```python
from build123d import *

# Parameters (mm, degrees)
EXTRUDE_1_DEPTH       = 2
HOLE_WIZARD_4_0_4_1_D = 4
HOLE_WIZARD_4_0_4_2_D = 4
FILLET_1_R            = 5
FILLET_2_R            = 5


with BuildPart() as part:
    # 草圖1 → 填料-伸長1 (new body)
    with BuildSketch(Plane(origin=(0, 0, 0), x_dir=(1, 0, 0), z_dir=(0, 1, 0))):
        Polygon((-28, -38), (-28, -58), (-10, -58), (-10, -96), (10, -96), (10, -58), (28, -58), (28, -38), (10, -38), (10, 0), (-10, 0), (-10, -38), align=None)
    extrude(amount=-EXTRUDE_1_DEPTH)

    # Ø4.0 (4) 直徑孔1 (through all)
    with Locations(Plane(origin=(0, 0, 0), x_dir=(1, 0, 0), z_dir=(0, 1, 0))):
        with Locations((0, -28), (0, -48), (0, -68), (0, -88), (-20, -48), (20, -48), (0, -8)):
            Hole(HOLE_WIZARD_4_0_4_1_D / 2)

    # Ø4.0 (4) 直徑孔2 (through all)
    with Locations(Plane(origin=(0, 0, 0), x_dir=(1, 0, 0), z_dir=(0, 1, 0))):
        with Locations((0, -18), (10, -48), (-10, -48), (0, -78)):
            Hole(HOLE_WIZARD_4_0_4_2_D / 2)

    # 圓角1
    fillet_1_edges = [part.edges().sort_by_distance(p)[0] for p in [
        (10, -1, 38),
        (10, -1, 58),
        (-10, -1, 58),
        (-10, -1, 38),
    ]]
    fillet(fillet_1_edges, radius=FILLET_1_R)

    # 圓角2
    fillet_2_edges = [part.edges().sort_by_distance(p)[0] for p in [
        (10, -1, 0),
        (28, -1, 38),
        (28, -1, 58),
        (10, -1, 96),
        (-10, -1, 96),
        (-28, -1, 58),
        (-28, -1, 38),
        (-10, -1, 0),
    ]]
    fillet(fillet_2_edges, radius=FILLET_2_R)


solid = part.part
```
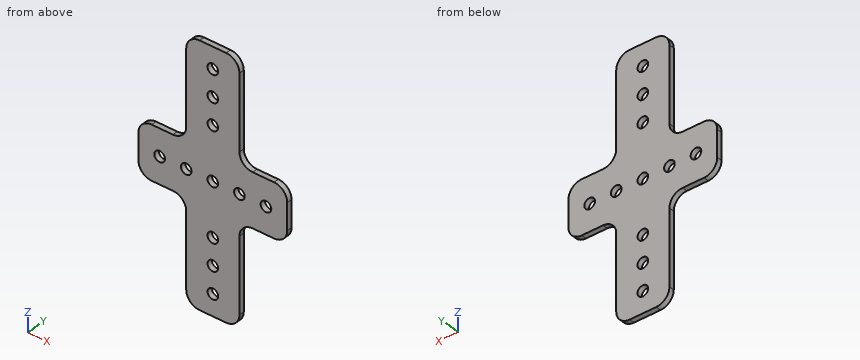
Can you work these out from the model? Positions are in its coordinate system, mm. Round coordinates to 2 decimals unless told otherwise and drop trailing zeros. Order: outer loops, then holes, each group sorted by start corner. A loop starts at its lowest first (then second) coordinate and runs counter-clockwise, first axis right, second up. Notation, with made-up numbers: (7, 59) -> (35, 59) arc R32 cw to (35, 87) -> close; hole circle Ø6 at (45.5, 88). An arc over 180 degrees is marked (long way). Return JSON: item names as keys, results as strings. Group by question number.
1. If we section it at B-B, the plane z = 8: Write out the boundary of the cut face in (x, y).
2. If we section it at C-C, the plane z = 48: Write out the boundary of the cut face in (x, y).
3. Will these pins go through, and if not, where does the flat tip stop? pin 1 (1 mm diameter, centred on y = -1, z = 20, fed in from -X); pin 2 (3 mm diameter, centred on x = 0, z = 8, fed in from +Y); pin 3 (0.6 mm diameter, centred on x = -18, y = -1.5, fed in from +Z); pin 4 (1 mm diameter, centred on x = -17, y = -1.5, fed in from -Z).
4. I need wall thicknesses on line 1 (X direction, y = -0.65, z = 48); line 2 (Z direction, x = 20, y = -0.85); line 3 (X direction, y = -0.5, z = 64). Which ranges of each line are inside material? Lowest first, please. Write a range as [from, to].
5. If we section it at A-A, the plane x = -20: Write out the boundary of the cut face in (y, z), then the cut area to 3 significant figures.
6. If we section it at D-D, the plane y = -1.4: Count the separate pieces of the cut face and the enclosed holes in it, then the cut area to 3 significant figures.
Output values:
{
 "1": {"outline": "(-10, -2) -> (-2, -2) -> (-2, 0) -> (-10, 0) -> close; (2, -2) -> (10, -2) -> (10, 0) -> (2, 0) -> close"},
 "2": {"outline": "(-28, -2) -> (-22, -2) -> (-22, 0) -> (-28, 0) -> close; (-18, -2) -> (-12, -2) -> (-12, 0) -> (-18, 0) -> close; (-8, -2) -> (-2, -2) -> (-2, 0) -> (-8, 0) -> close; (2, -2) -> (8, -2) -> (8, 0) -> (2, 0) -> close; (12, -2) -> (18, -2) -> (18, 0) -> (12, 0) -> close; (22, -2) -> (28, -2) -> (28, 0) -> (22, 0) -> close"},
 "3": {"pin 1": "x = -10", "pin 2": "through", "pin 3": "z = 58", "pin 4": "z = 38"},
 "4": {"line 1": "[-28, -22], [-18, -12], [-8, -2], [2, 8], [12, 18], [22, 28]", "line 2": "[38, 46], [50, 58]", "line 3": "[-10, 10]"},
 "5": {"outline": "(-2, 38) -> (0, 38) -> (0, 46) -> (-2, 46) -> close; (-2, 50) -> (0, 50) -> (0, 58) -> (-2, 58) -> close", "area": "32.0 mm²"},
 "6": {"separate pieces": "1", "enclosed holes": "11", "area": "2,480 mm²"}
}
